Autodesk Inventor part; units mm, degrees
ref_plane "YZ Plane" through (0, 0, 0) normal (1, 0, 0) x (0, 1, 0)
ref_plane "XZ Plane" through (0, 0, 0) normal (0, 1, 0) x (-1, 0, 0)
ref_plane "XY Plane" through (0, 0, 0) normal (0, 0, 1) x (1, 0, 0)
sketch "Sketch1" plane through (0, 0, 0) normal (0, 0, 1) x (1, 0, 0)
  line L0 (45, -50) -> (25, -50)
  line L1 (-45, -50) -> (-45, 50)
  line L2 (-45, 50) -> (-25, 50)
  line L3 (45, 50) -> (45, -50)
  line L4 (45, -50) -> (-45, 50) construction
  line L5 (-45, -50) -> (45, 50) construction
  line L6 (-25, 50) -> (25, 50) construction
  line L7 (25, 50) -> (25, 54)
  line L8 (25, 54) -> (-25, 54)
  line L9 (-25, 54) -> (-25, 50)
  line L10 (-25, -50) -> (25, -50) construction
  line L11 (25, -50) -> (25, -54)
  line L12 (25, -54) -> (-25, -54)
  line L13 (-25, -54) -> (-25, -50)
  line L14 (-45, 50) -> (-49, 50)
  line L15 (-49, 50) -> (-49, 25)
  line L16 (-49, 25) -> (-45, 25)
  line L17 (-45, 25) -> (-45, 50)
  line L18 (-45, 0) -> (-45, 25)
  line L19 (-45, 25) -> (-49, 25)
  line L20 (-49, 25) -> (-49, 0)
  line L21 (-49, 0) -> (-45, 0)
  line L22 (-45, -25) -> (-45, 0) construction
  line L23 (-45, 0) -> (-49, 0)
  line L24 (-49, 0) -> (-49, -25)
  line L25 (-49, -25) -> (-45, -25)
  line L26 (-45, -50) -> (-45, -25)
  line L27 (-45, -25) -> (-49, -25)
  line L28 (-49, -25) -> (-49, -50)
  line L29 (-49, -50) -> (-45, -50)
  line L30 (0, -75.6) -> (0, 75.6)
  line L31 (45, 20) -> (49, 20)
  line L32 (49, 20) -> (49, -20)
  line L33 (49, -20) -> (45, -20)
  line L34 (45, -20) -> (45, 20)
  line L35 (25, 50) -> (45, 50)
  line L36 (-25, 50) -> (25, 50) construction
  line L37 (-25, -50) -> (-45, -50)
  line L38 (25, -50) -> (-25, -50)
  line L39 (-68.6, 0) -> (68.6, 0)
  point P0 (0, 0)
  dimension "d0" = 90
  dimension "d1" = 100
  dimension "d2" = 50
  dimension "d3" = 4
  dimension "d4" = 50
  dimension "d5" = 4
  dimension "d6" = 4
  dimension "d7" = 25
  dimension "d10" = 25
  dimension "d17" = 4
  dimension "d18" = 40
extrude "Extrusion1" add sketch "Sketch1" along normal blind 4 contours L0 L38 L30 L39 L3 | L11 L12 L30 L38 | L3 L39 L32 L33 | L38 L37 L1 L39 L30 | L30 L12 L13 L38 | L39 L30 L8 L7 L35 L3 | L3 L31 L32 L39 | L39 L1 L2 L9 L8 L30 | L1 L25 L24 L21 | L16 L15 L14 L1
properties part number "CarSide_V1" material "Wood (Oak)"
CAD build for the part. Positions are in the model's coordinates, mm. A direction names the side the tool comes from. Give positions to 0.01 mm unless a question says otherwise; leave off trailing zeros. Loops run counter-clockwise (first coordinate to the right, second up) from the corner with the lowest first, then second, coordinate; pieces in that order, holes last. Notation, with made-up numbers: M 64,68.5 L 75,68.5 A14 cw 75,92.5 Z; hole C 46,-8.5 d8. An arc over 180 degrees is marked long. Use one line per item in the form item = value.
Item 1: Slice it at C-C (x = -26.5). List the corners of the cut face in (y, z), plus the area to 3 significant figures.
Determined:
outline = M -50,0 L 50,0 L 50,4 L -50,4 Z
area = 400 mm2
Item 2: Flat gauge pins, fed straight in: pin 1 (1.2 mm diameter, centred on x = -46.5, z = 1, fed in from +Y); pin 2 (2 mm diameter, centred on x = -47.5, z = 2.5, fed in from -Y); pin 3 (5 mm diameter, centred on x = -31, y = 11, fed in from -Z); pin 4 (2 mm diameter, centred on x = -30.5, z = 2, fed in from -Y). Where does each tip first touch, or does it go through?
Determined:
pin_1 = 50
pin_2 = -25
pin_3 = 0
pin_4 = -50
Item 3: Slice it at A-A (z = 3.15). List the corners of the cut face in (x, y), plus the area to 3 significant figures.
Determined:
outline = M -49,-25 L -45,-25 L -45,-50 L -25,-50 L -25,-54 L 25,-54 L 25,-50 L 45,-50 L 45,-20 L 49,-20 L 49,20 L 45,20 L 45,50 L 25,50 L 25,54 L -25,54 L -25,50 L -49,50 L -49,25 L -45,25 L -45,0 L -49,0 Z
area = 9,760 mm2
Item 4: Drill centre lines: probe 1 along X at (y, z) = (42, 1.8); probe 2 along X at (y, z) = (-48, 0.95); probe 3 along Y at (x, z) = (43, 1). Where is each one in solid material? Low to high. Write a range as from..to.
Determined:
probe_1 = -49..45
probe_2 = -45..45
probe_3 = -50..50
Item 5: Which spindle directions (+Z, -Z, +X, -X, +Y, -Y) get a long thin tool onto all of the face, cutting with end or side? Do faces 4 (the face through (47, -20, 2)), 5 (the face through (-45, -38, 2)), 6 (the face through (-37, 50, 2)), 7 (the face through (47, 20, 2)). Say none if no direction does.
Determined:
face_4 = +Z, -Z, +X, -Y
face_5 = +Z, -Z, -X, -Y
face_6 = +Z, -Z, -X, +Y
face_7 = +Z, -Z, +X, +Y
Item 6: Slice it at B-B (y = 34). List the corners of the cut face in (x, z).
Determined:
outline = M -49,0 L 45,0 L 45,4 L -49,4 Z
Item 7: Two-plate mould, pull along Y, no slides. Class faces 1 (the face through (0, -54, 2)), 2 (the face through (-45, 12, 2)), 3 (the face through (-25, -52, 2)): pulls with the +Y half, pulls with the -Y half, needs draft (parallel to the pull), parting line crosses it, or undercut.
Determined:
face_1 = pulls with the -Y half
face_2 = undercut
face_3 = needs draft
